Print and shaded views of the part. All mm, measured from the part's lowest x, y and z. Round coordinates to 2 decimals unless told otherwise and drop trailing zeros. Write each loop counter-clockwise with the first axis right and the second up, starting at its lowest first coordinate (ties: lowest second). Pieces come first, ordered by that corner, then holes. Notation, with made-up numbers: (-26.75, -28.5) -> (11.25, -28.5) arc R18 cw to (11.25, -21.5) -> close; hole circle Ø11 at (52.25, 83.5). An arc over 180 degrees is marked (long way). Return JSON: item names as keys, results as strings. Group by question number.
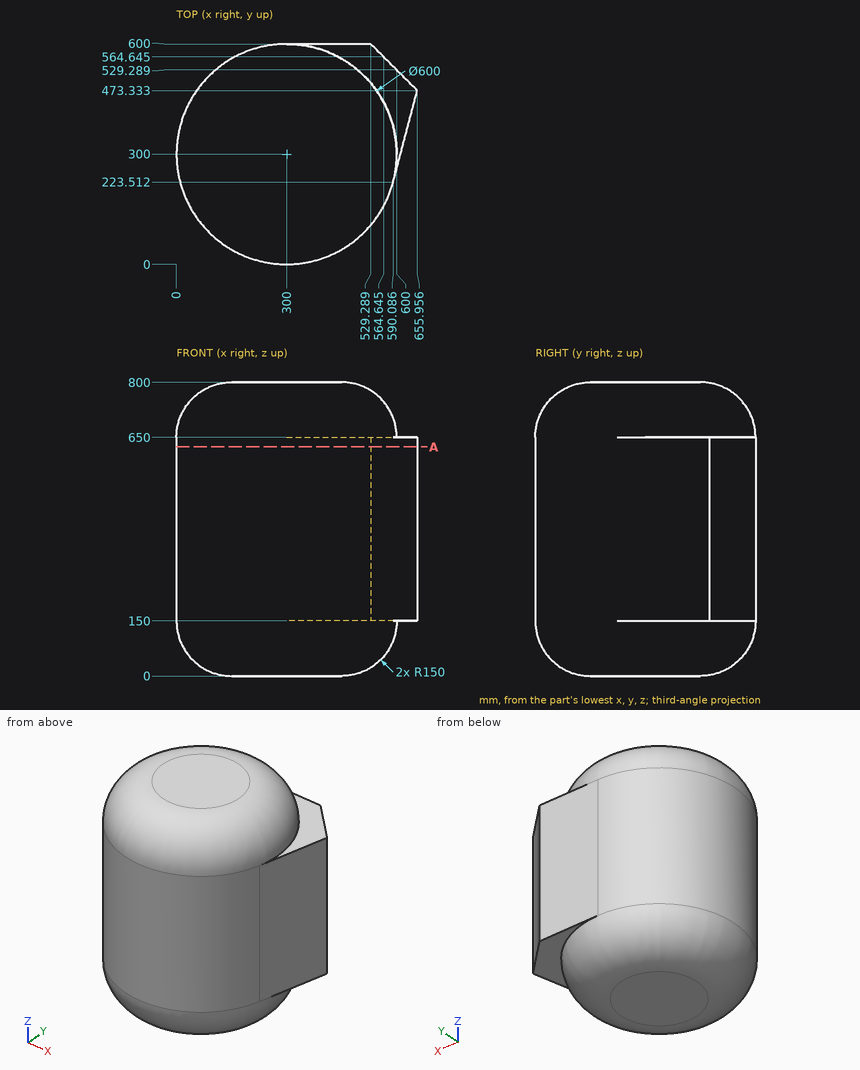
Item 1: Wall check: L1, parallel to Y at x = 123, z = 268; L2, parallel to X at y = 42, z = 449.5 (1 decimal); L3, parallel to Y at x = 240, z = 417.5. Give the ranges that are in metal, low to high.
Item 2: Flat gauge pins, fed straight in: P1, Ø10, axis at x = 357.5, y = 483, coming from the +Z side; P2, Ø2, axis at x = 485, y = 85.5, coming from the -Z side (1 decimal); P3, Ø2, axis at x = 84, z = 645.5, coming from the -Y side (1 decimal); P4, Ø10, axis at x = 304, y = 356, coming from the -Z side. Where does each tip first touch, or does it go through?
Item 3: Cut at A-A (z = 624). Write the cut outline in (x, y) (1 decimal).
Checks:
{
 "1": {"L1": "y = 57.78 to 542.22", "L2": "x = 146.9 to 453.1", "L3": "y = 6.06 to 593.94"},
 "2": {"P1": "stops at z = 795.41", "P2": "stops at z = 79.2", "P3": "stops at y = 90.8", "P4": "stops at z = 0"},
 "3": {"outline": "(300, 600) arc R300 ccw (long way) to (590.1, 223.5) -> (656, 473.3) -> (529.3, 600) -> close"}
}
